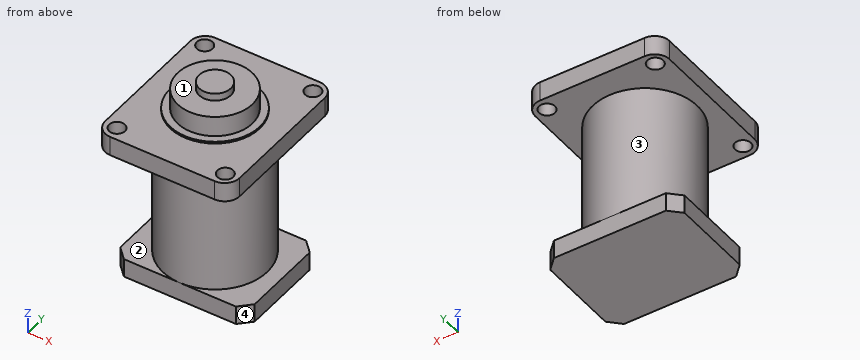
```python
from build123d import *

# Parameters (mm, degrees)
F0_R      = 26.9875
F1_DEPTH  = 66.675
F2_R      = 152.4
F3_DEPTH  = 6.35
F4_R      = 127
F5_DEPTH  = 76.2
F6_R      = 53.975
F7_DEPTH  = 25.4
F8_R      = 177.8
F9_DEPTH  = 508
F10_W     = 457.2
F10_H     = 355.6
F11_DEPTH = 63.5
F12_SIZE  = 38.1


with BuildPart() as f1:
    # F0 (on Top) → F1 (new body)
    with BuildSketch(Plane.XY):
        with BuildLine():
            Line((177.8, 266.7), (-177.8, 266.7))
            ThreePointArc((-177.8, 266.7), (-213.721024, 251.821024), (-228.6, 215.9))
            Line((-228.6, 215.9), (-228.6, -215.9))
            ThreePointArc((-228.6, -215.9), (-213.721024, -251.821024), (-177.8, -266.7))
            Line((-177.8, -266.7), (177.8, -266.7))
            ThreePointArc((177.8, -266.7), (213.721024, -251.821024), (228.6, -215.9))
            Line((228.6, -215.9), (228.6, 215.9))
            ThreePointArc((228.6, 215.9), (213.721024, 251.821024), (177.8, 266.7))
        make_face()
        with Locations((-184.15, -222.25)):
            Circle(F0_R, mode=Mode.SUBTRACT)
        with Locations((184.15, -222.25)):
            Circle(F0_R, mode=Mode.SUBTRACT)
        with Locations((-184.15, 222.25)):
            Circle(F0_R, mode=Mode.SUBTRACT)
        with Locations((184.15, 222.25)):
            Circle(F0_R, mode=Mode.SUBTRACT)
    extrude(amount=F1_DEPTH)

    # F2 (on face) → F3 (join)
    with BuildSketch(Plane.XY.offset(66.675)):
        Circle(F2_R)
    extrude(amount=F3_DEPTH)

    # F4 (on face) → F5 (join)
    with BuildSketch(Plane.XY.offset(66.675)):
        Circle(F4_R)
    extrude(amount=F5_DEPTH)

    # F6 (on face) → F7 (join)
    with BuildSketch(Plane.XY.offset(142.875)):
        Circle(F6_R)
    extrude(amount=F7_DEPTH)

    # F8 (on face) → F9 (join)
    with BuildSketch(Plane(origin=(0, 0, 0), x_dir=(1, 0, 0), z_dir=(0, 0, -1))):
        Circle(F8_R)
    extrude(amount=F9_DEPTH)

    # F10 (on face) → F11 (join)
    with BuildSketch(Plane(origin=(0, 0, -508), x_dir=(1, 0, 0), z_dir=(0, 0, -1))):
        Rectangle(F10_W, F10_H)
    extrude(amount=-F11_DEPTH)

    # F12
    f12_edges = [f1.edges().sort_by_distance(p)[0] for p in [
        (228.6, -177.8, -476.25),
        (-228.6, -177.8, -476.25),
        (228.6, 177.8, -476.25),
        (-228.6, 177.8, -476.25),
    ]]
    chamfer(f12_edges, length=F12_SIZE)


solid = f1.part
```
For this review, take the finished solid that the model builds, in its own axes (mm). Face numbers are marked on the shaded views. A direction names the side the tool comes from. Round coordinates to 2 decimals unless told otherwise and drop trailing zeros. Write each loop counter-clockwise with the first axis right and the second up, starting at its lowest first coordinate (ties: lowest second). Pieces come first, ordered by that corner, then holes. Notation, with made-up numbers: (-21, 72) - (-3, 72) arc R14 ccw to (-3, 77) - close; hole circle Ø8 at (-20.5, 28). An arc over 180 degrees is marked (long way). Answer as a JSON object with one key per item and string values.
1. We need section C-C on z = -385. Give the boundary of the cut face in (x, y).
Response values:
{"outline": "circle Ø355.6 at (0, 0)"}
2. For pin 1 Ø12 at (y, z) = (-44.5, -237.5) entering from -X; pin 2 Ø6 at (x, z) = (14, 92) entering from +Y; pin 3 Ø5 at (x, z) = (53.5, -3) entering from +Y, all flat-tipped, find the tip position at first contact; note any pin that passes through.
Response values:
{"pin 1": "stops at x = -173.58", "pin 2": "stops at y = 126.52", "pin 3": "stops at y = 170.33"}
3. To check wall thickness, follow line 1 along Y through (x, z) = (-184.15, 34.5); line 2 along Z through (x, y) = (-174, 154) (3 decimals); line 3 along Z through (x, y) = (-134, 63) (3 decimals). State the ranges of each line that lie inside material, in increasing order.
Response values:
{"line 1": "y = -266.3 to -249.24, -195.26 to 195.26, 249.24 to 266.3", "line 2": "z = -508 to -444.5, 0 to 66.675", "line 3": "z = -508 to 73.025"}
4. Tool access review of the marked faces 1, 2, 3 and 4: name each direction out of +Z, -Z, +X, -X, +Y, -Y from which nothing blocks a thin tool from reaching the whole face with its end or side.
Response values:
{"face 1": "+Z", "face 2": "-X", "face 3": "none", "face 4": "-Z, +X, -Y"}
5. We need section A-A on y = 0. Give the boundary of the cut face in (x, z) (3 decimals), then the cut area to 3 significant figures.
Response values:
{"outline": "(-228.6, -508) - (228.6, -508) - (228.6, -444.5) - (177.8, -444.5) - (177.8, 0) - (228.6, 0) - (228.6, 66.675) - (152.4, 66.675) - (152.4, 73.025) - (127, 73.025) - (127, 142.875) - (53.975, 142.875) - (53.975, 168.275) - (-53.975, 168.275) - (-53.975, 142.875) - (-127, 142.875) - (-127, 73.025) - (-152.4, 73.025) - (-152.4, 66.675) - (-228.6, 66.675) - (-228.6, 0) - (-177.8, 0) - (-177.8, -444.5) - (-228.6, -444.5) - close", "area": "240,000 mm2"}
6. We need section B-B on x = -28. Give the boundary of the cut face in (y, z) (3 decimals).
Response values:
{"outline": "(-266.7, 0) - (-175.581, 0) - (-175.581, -444.5) - (-177.8, -444.5) - (-177.8, -508) - (177.8, -508) - (177.8, -444.5) - (175.581, -444.5) - (175.581, 0) - (266.7, 0) - (266.7, 66.675) - (149.806, 66.675) - (149.806, 73.025) - (123.875, 73.025) - (123.875, 142.875) - (46.144, 142.875) - (46.144, 168.275) - (-46.144, 168.275) - (-46.144, 142.875) - (-123.875, 142.875) - (-123.875, 73.025) - (-149.806, 73.025) - (-149.806, 66.675) - (-266.7, 66.675) - close"}
7. We need section D-D on y = 93. Give the boundary of the cut face in (x, z) (3 decimals).
Response values:
{"outline": "(-228.6, -508) - (228.6, -508) - (228.6, -444.5) - (151.538, -444.5) - (151.538, 0) - (228.6, 0) - (228.6, 66.675) - (120.734, 66.675) - (120.734, 73.025) - (86.487, 73.025) - (86.487, 142.875) - (-86.487, 142.875) - (-86.487, 73.025) - (-120.734, 73.025) - (-120.734, 66.675) - (-228.6, 66.675) - (-228.6, 0) - (-151.538, 0) - (-151.538, -444.5) - (-228.6, -444.5) - close"}
